Autodesk Inventor part; units mm, degrees
ref_plane "YZ Plane" through (0, 0, 0) normal (1, 0, 0) x (0, 1, 0)
ref_plane "XZ Plane" through (0, 0, 0) normal (0, 1, 0) x (-1, 0, 0)
ref_plane "XY Plane" through (0, 0, 0) normal (0, 0, 1) x (1, 0, 0)
sketch "Эскиз1" plane through (0, 0, 0) normal (0, 0, 1) x (1, 0, 0)
  circle A0 centre (15, 10.75) radius 1.75
  circle A1 centre (-15, 10.75) radius 1.75
  circle A2 centre (-15, -10.75) radius 1.75
  circle A3 centre (15, -10.75) radius 1.75
  arc A4 (15, 6.75) -> (15, 14.75) centre (15, 10.75) ccw
  arc A5 (15, -14.75) -> (15, -6.75) centre (15, -10.75) ccw
  arc A6 (-15, 14.75) -> (-15, 6.75) centre (-15, 10.75) ccw
  arc A7 (-15, -6.75) -> (-15, -14.75) centre (-15, -10.75) ccw
  line L0 (15, 14.75) -> (12, 14.75)
  line L1 (12, 14.75) -> (12, -14.75)
  line L2 (12, -14.75) -> (15, -14.75)
  line L3 (15, -6.75) -> (15, 6.75)
  line L4 (-15, 14.75) -> (-12, 14.75)
  line L5 (-12, 14.75) -> (-12, -14.75)
  line L6 (-12, -14.75) -> (-15, -14.75)
  line L7 (-15, -6.75) -> (-15, 6.75)
  point P0 (0, 0)
  dimension "d0" = 3
extrude "Выдавливание1" add sketch "Эскиз1" along normal blind 11
sketch "Эскиз2" plane through (-12, -14.75, 0) normal (1, 0, 0) x (0, 0, -1)
  line L0 (-11, 0) -> (-11, 29.5)
  line L1 (-11, 29.5) -> (-5, 29.5)
  line L2 (-5, 0) -> (-11, 0)
  line L3 (-11, 0) -> (-11, 29.5)
  line L4 (0, 0) -> (-11, 0)
  arc A0 (-11, 8) -> (-11, 22) centre (-11, 15) ccw
  point P0 (0, 14.75)
  dimension "d4" = 6
  dimension "d5" = 7
  dimension "d13" = 14.5
extrude "Выдавливание2" cut sketch "Эскиз2" along normal blind 30 and the other way blind 6
sketch "Эскиз3" plane through (0, 0, 0) normal (0, 0, -1) x (-1, 0, 0)
  line L0 (12, 14.75) -> (12, -14.75)
  line L1 (-12, -2.5) -> (12, -2.5)
  line L2 (12, -2.5) -> (12, 2.5)
  line L3 (12, 2.5) -> (-12, 2.5)
  line L4 (-12, 2.5) -> (-12, -2.5)
  line L5 (-12, -2.5) -> (12, 2.5) construction
  line L6 (12, -2.5) -> (-12, 2.5) construction
  point P0 (0, 0)
  dimension "d10" = 5
extrude "Выдавливание3" add sketch "Эскиз3" against normal blind 2
sketch "Эскиз5" plane through (0, 0, 11) normal (0, 0, 1) x (1, 0, 0)
  circle A0 centre (15, -10.75) radius 1.75
  line L0 (15, -6.75) -> (12, -6.75)
  line L1 (12, -6.75) -> (12, -14.75)
  line L2 (12, -14.75) -> (15, -14.75)
  arc A1 (15, -14.75) -> (15, -6.75) centre (15, -10.75) ccw
  line L3 (12, -6.75) -> (15, -6.75)
  line L4 (15, -6.75) -> (15, -2.5)
  line L5 (15, -2.5) -> (12, -2.5)
  line L6 (12, -2.5) -> (12, -6.75)
  point P0 (0, 0)
extrude "Выдавливание4" cut sketch "Эскиз5" against normal blind 2
sketch "Эскиз6" plane through (0, 0, 9) normal (0, 0, 1) x (1, 0, 0)
  line L0 (-25, 4) -> (25, 4)
  line L1 (25, 4) -> (25, -4)
  line L2 (25, -4) -> (-25, -4)
  line L3 (-25, -4) -> (-25, 4)
  line L4 (-25, 4) -> (25, -4) construction
  line L5 (25, 4) -> (-25, -4) construction
  circle A0 centre (15, -10.75) radius 1.75
  circle A1 centre (15, -10.75) radius 6
  point P0 (0, 0)
  dimension "d19" = 50
  dimension "d20" = 8
  dimension "d21" = 12
properties part number "Fastening"
Input: part model. Units: mm. Frame: model coordinates. A direction names the side the tool comes from. Give positions to 0.01 mm unless a question says otherwise; leave off trailing zeros. Loops run counter-clockwise (first coordinate to the right, second up) from the corner with the lowest first, then second, coordinate; pieces in that order, holes last. Notation, with made-up numbers: (75, 21) -> (130, 21) arc R22 ccw to (130, 31) -> close; hole circle Ø8 at (21.25, 88.25). An arc over 180 degrees is marked (long way). Use a Markdown table: item, result.
Q1. First-contact query: P1, Ø10, axis at x = -4, y = 4.5, coming from the -Z side; P2, Ø5.5, axis at y = -2.5, z = 6.5, coming from the +X side; P3, Ø3.5, axis at y = -3, z = 4, coming from the -X side; P4, Ø1, axis at x = 3, z = 1, coming from the -Y side. Flat tips, straight axial feed; report the tip coordinate or a pass-through.
Entries:
| item | result |
|---|---|
| P1 | stops at z = 0 |
| P2 | stops at x = 15 |
| P3 | stops at x = -15 |
| P4 | stops at y = -2.5 |
Q2. Access query for faces 4 (the flat face through (-13, -14.75, 5)), 5 (the cylindrical face through (13.885, 1.399, 4.095)), 6 (the flat face through (0, 0, 2)), 7 (the flat face through (15, 0, 2)), 8 (the flat face through (0, 2.5, 1)). Directions: +Z, -Z, +X, -X, +Y, -Y. A direction counts if a zero-diameter tool reaches every point of the face in a straight line with its end or side. Return the directions, or none.
Entries:
| item | result |
|---|---|
| face 4 | +Z, -Z, +X, -X, -Y |
| face 5 | +Z, +X, -X |
| face 6 | +Z, +Y, -Y |
| face 7 | +Z, -Z, +X |
| face 8 | +Z, -Z, +Y |
Q3. Ray query, probe 1 along X at (y, z) = (6.5, 2.25); probe 2 along Z at (x, y) = (3.5, -2.25); probe 3 along Y at (x, z) = (-0.5, 1.75). Return the intervals inside material, ascending. Write a range as from..to.
Entries:
| item | result |
|---|---|
| probe 1 | x = -15..-12, 12..15 |
| probe 2 | z = 0..2 |
| probe 3 | y = -2.5..2.5 |
Q4. Section query B-B, the plane y = -10.75. Return the cut outline in (x, z), plus the area to 3 significant figures.
Entries:
| item | result |
|---|---|
| outline | (-19, 0) -> (-16.75, 0) -> (-16.75, 11) -> (-19, 11) -> close; (-13.25, 0) -> (-12, 0) -> (-12, 11) -> (-13.25, 11) -> close; (12, 0) -> (13.25, 0) -> (13.25, 9) -> (12, 9) -> close; (16.75, 0) -> (19, 0) -> (19, 9) -> (16.75, 9) -> close |
| area | 70.0 mm² |
Q5. Section query C-C, the plane y = 3. Return the cut outline in (x, z), plus the area to 3 significant figures.
Entries:
| item | result |
|---|---|
| outline | (-15, 0) -> (-12, 0) -> (-12, 4.56) -> (-15, 4.56) -> close; (12, 0) -> (15, 0) -> (15, 4.56) -> (12, 4.56) -> close |
| area | 27.4 mm² |
Q6. Section query D-D, the plane z = 9.75. Return the cut outline in (x, y), plus the area to 3 significant figures.
Entries:
| item | result |
|---|---|
| outline | (-16.72, 7.14) -> (-12, 7.14) -> (-12, 14.75) -> (-15, 14.75) arc R4 ccw to start; (-15, -14.75) -> (-12, -14.75) -> (-12, -6.64) -> (-15, -6.64) -> (-15, -6.75) arc R4 ccw to start; (12, 7.14) -> (16.72, 7.14) arc R4 ccw to (15, 14.75) -> (12, 14.75) -> close; hole circle Ø3.5 at (-15, -10.75); hole circle Ø3.5 at (-15, 10.75); hole circle Ø3.5 at (15, 10.75) |
| area | 116 mm² |
Q7. Section query A-A, the plane z = 3.5. Return the cut outline in (x, y), plus the area to 3 significant figures.
Entries:
| item | result |
|---|---|
| outline | (-15, -14.75) -> (-12, -14.75) -> (-12, 14.75) -> (-15, 14.75) arc R4 ccw to (-15, 6.75) -> (-15, -6.75) arc R4 ccw to start; (12, -14.75) -> (15, -14.75) arc R4 ccw to (15, -6.75) -> (15, 6.75) arc R4 ccw to (15, 14.75) -> (12, 14.75) -> close; hole circle Ø3.5 at (-15, -10.75); hole circle Ø3.5 at (-15, 10.75); hole circle Ø3.5 at (15, -10.75); hole circle Ø3.5 at (15, 10.75) |
| area | 239 mm² |
Q8. Pull-direction query (Y, two-part tool) for faces 1 (the flat face through (0, -2.5, 1)), 2 (the cylindrical face through (-14.059, -12.226, 5.423)), 3 (the flat face through (-16, 13, 11)); classes: pulls with the +Y half, pulls with the -Y half, needs draft (parallel to the pull), parting line crosses it, or undercut.
Entries:
| item | result |
|---|---|
| face 1 | pulls with the -Y half |
| face 2 | undercut |
| face 3 | needs draft |
